from build123d import *

# Parameters (mm, degrees)
SKETCH1_W           = 24
SKETCH1_H           = 120
BOSS_EXTRUDE1_DEPTH = 50
SKETCH3_R           = 6
CUT_EXTRUDE1_DEPTH  = 133.196822957
SKETCH5_R           = 5
CUT_EXTRUDE4_DEPTH  = 133.196822957
SKETCH4_W           = 18
SKETCH4_H           = 80
CUT_EXTRUDE5_DEPTH  = 133.196822957
CUT_EXTRUDE7_START  = -24
CUT_EXTRUDE7_DEPTH  = 24
FILLET2_R           = 1


# Read off the part's stored shape, not the designer's step: Cut-Extrude7
with BuildPart() as part:
    # Sketch1 → Boss-Extrude1 (new body)
    with BuildSketch(Plane(origin=(0, 0, 0), x_dir=(0, 0, -1), z_dir=(1, 0, 0))):
        with Locations((-12, -60)):
            Rectangle(SKETCH1_W, SKETCH1_H)
    extrude(amount=BOSS_EXTRUDE1_DEPTH)

    # Sketch3 → Cut-Extrude1 (cut, through all)
    with BuildSketch(Plane.XY.offset(24)):
        with Locations((25, -25)):
            Circle(SKETCH3_R)
    extrude(amount=-CUT_EXTRUDE1_DEPTH, mode=Mode.SUBTRACT)

    # Sketch5 → Cut-Extrude4 (cut, through all)
    with BuildSketch(Plane.XY.offset(24)):
        with Locations((25, -120)):
            Circle(SKETCH5_R)
    extrude(amount=-CUT_EXTRUDE4_DEPTH, mode=Mode.SUBTRACT)

    # Sketch4 → Cut-Extrude5 (cut, through all)
    with BuildSketch(Plane(origin=(50, 0, 0), x_dir=(0, 0, -1), z_dir=(1, 0, 0))):
        with Locations((-12, -120)):
            Rectangle(SKETCH4_W, SKETCH4_H)
    extrude(amount=-CUT_EXTRUDE5_DEPTH, mode=Mode.SUBTRACT)

    # Cut-Extrude7 outline → Cut-Extrude7 (cut)
    with BuildSketch(Plane.XY.offset(24).offset(CUT_EXTRUDE7_START)):
        with BuildLine():
            Line((0, 0), (0, -25))
            ThreePointArc((0, -25), (7.32233047, -7.32233047), (25, 0))
            Line((25, 0), (0, 0))
        make_face()
        with BuildLine():
            Line((50, 0), (25, 0))
            ThreePointArc((25, 0), (42.67766953, -7.32233047), (50, -25))
            Line((50, -25), (50, 0))
        make_face()
    extrude(amount=CUT_EXTRUDE7_DEPTH, mode=Mode.SUBTRACT)

    # Fillet2
    fillet2_edges = [part.edges().sort_by_distance(p)[0] for p in [
        (19, -25, 0),
    ]]
    fillet(fillet2_edges, radius=FILLET2_R)


solid = part.part
Verification items for the finished model (mm, model axes). A direction names the side the tool comes from. Give positions to 0.01 mm unless a question says otherwise; leave off trailing zeros. Loops run counter-clockwise (first coordinate to the right, second up) from the corner with the lowest first, then second, coordinate; pieces in that order, holes last. Notation, with made-up numbers: (25.5, 67.5) - (80.5, 67.5) arc R22 ccw to (80.5, 79.5) - close; hole circle Ø4 at (-23, 49.25). An arc over 180 degrees is marked (long way). Write each question's results on one line, items separated by ' | '.
1) Sectioned sample at A-A on y = -101. Record the boundary of the cut face in (x, z).
Solution:
outline: (0, 0) - (50, 0) - (50, 3) - (0, 3) - close; (0, 21) - (50, 21) - (50, 24) - (0, 24) - close
2) Depth check by flat-ended pin: P1, Ø2, axis at x = 8, z = 19.5, coming from the -Y side; P2, Ø7, axis at x = 25, y = -25, coming from the -Z side; P3, Ø12, axis at x = 17.5, y = -93.5, coming from the -Z side; P4, Ø5, axis at x = 10, z = 3.5, coming from the +Y side. Enter the tip coordinate at first touch or a pass-through.
Solution:
P1: y = -80 | P2: through | P3: z = 0 | P4: y = -3.35
3) Tool access check on faces 4 (the flat face through (25, -80, 12)), 5 (the flat face through (0, -61, 12)). Record the directions out of +Z, -Z, +X, -X, +Y, -Y that give a thin tool (end or side, any length) a straight path to the whole face; none if there is none.
Solution:
face 4: +X, -X, -Y | face 5: +Z, -Z, -X, +Y, -Y
4) Material ranges on L1, parallel to Z at x = 35.5, y = -81; L2, parallel to Y at x = 25, z = 8.25; L3, parallel to Y at x = 26, z = 13.75, recorded low to high. Write a range as from..to.
Solution:
L1: 0..3, 21..24 | L2: -80..-31, -19..0 | L3: -80..-30.92, -19.08..-0.02
5) Mould release check, pull along Y, two halves, no side actions. Record for faces 1 (the cylindrical face through (25, -115, 2)), 2 (the cylindrical face through (20.24, -28.65, 12.66)), 3 (the flat face through (25, -61, 24)): pulls with the +Y half, pulls with the -Y half, needs draft (parallel to the pull), parting line crosses it, or undercut.
Solution:
face 1: pulls with the -Y half | face 2: undercut | face 3: needs draft
6) Sectioned sample at D-D on x = 34. Record the boundary of the cut face in (y, z).
Solution:
outline: (-120, 0) - (-1.68, 0) - (-1.68, 24) - (-120, 24) - (-120, 21) - (-80, 21) - (-80, 3) - (-120, 3) - close
7) Sectioned sample at B-B on z = 9. Record the boundary of the cut face in (x, y).
Solution:
outline: (0, -80) - (50, -80) - (50, -25) arc R25 ccw to (0, -25) - close; hole circle Ø12 at (25, -25)
8) Sectioned sample at C-C on x = 40. Record the boundary of the cut face in (y, z), plus the area to 3 significant figures.
Solution:
outline: (-120, 0) - (-5, 0) - (-5, 24) - (-120, 24) - (-120, 21) - (-80, 21) - (-80, 3) - (-120, 3) - close | area: 2,040 mm2
